For this review, take the finished solid that the model builds, in its own axes (mm). A direction names the side the tool comes from. Coordinates: 2 decimals unless noted, no trailing zeros. Write each loop counter-clockwise with the first axis right and the second up, starting at its lowest first coordinate (ties: lowest second). Pieces come first, ordered by that corner, then holes.
```python
from build123d import *

# Parameters (mm, degrees)
SKETCH_1_W          = 110
SKETCH_1_H          = 100
EXTRUDE_1_DEPTH     = 20
SKETCH_2_R          = 31.25
CUT_EXTRUDE_1_DEPTH = 14
SKETCH_3_R          = 21.5
CUT_EXTRUDE_2_DEPTH = 14
SKETCH_4_R          = 1.65
CUT_EXTRUDE_3_DEPTH = 77.974021592


with BuildPart() as part:
    # 草图1 → 凸台-拉伸1 (new body)
    with BuildSketch(Plane(origin=(0, 0, 0), x_dir=(0, 0, -1), z_dir=(1, 0, 0))):
        Rectangle(SKETCH_1_W, SKETCH_1_H)
    extrude(amount=EXTRUDE_1_DEPTH)

    # 草图2 → 切除-拉伸1 (cut)
    with BuildSketch(Plane(origin=(20, 0, 0), x_dir=(0, 0, -1), z_dir=(1, 0, 0))):
        Circle(SKETCH_2_R)
    extrude(amount=-CUT_EXTRUDE_1_DEPTH, mode=Mode.SUBTRACT)

    # 草图3 → 切除-拉伸2 (cut)
    with BuildSketch(Plane(origin=(6, 0, 0), x_dir=(0, 0, -1), z_dir=(1, 0, 0))):
        Circle(SKETCH_3_R)
    extrude(amount=-CUT_EXTRUDE_2_DEPTH, mode=Mode.SUBTRACT)

    # 草图4 → 切除-拉伸3 (cut, through all)
    with BuildSketch(Plane(origin=(20, 0, 0), x_dir=(0, 0, -1), z_dir=(1, 0, 0))):
        with Locations((33, 40)):
            Circle(SKETCH_4_R)
        with Locations((11, 40)):
            Circle(SKETCH_4_R)
        with Locations((-11, 40)):
            Circle(SKETCH_4_R)
        with Locations((-33, 40)):
            Circle(SKETCH_4_R)
        with Locations(Location((-11, -40, 0), (0, 0, 180))):
            Circle(SKETCH_4_R)
        with Locations(Location((11, -40, 0), (0, 0, 180))):
            Circle(SKETCH_4_R)
        with Locations(Location((33, -40, 0), (0, 0, 180))):
            Circle(SKETCH_4_R)
        with Locations(Location((-33, -40, 0), (0, 0, 180))):
            Circle(SKETCH_4_R)
    extrude(amount=-CUT_EXTRUDE_3_DEPTH, mode=Mode.SUBTRACT)


solid = part.part
```
1) Consider section A-A (z = 33). Give the boundary of the cut face in (x, y), then the cut area to 3 significant figures.
2) Consider section D-D (z = 0). Give the boundary of the cut face in (x, y), then the cut area to 3 significant figures.
3) Tool access review of faces 1 (the face through (10.14, 41.39, 10.11)), 2 (the face through (13.1, 1.37, 31.22)): name each direction out of +Z, -Z, +X, -X, +Y, -Y from which nothing blocks a thin tool from reaching the whole face with its end or side.
4) For L1, parallel to Y at x = 6.75, z = -33; L2, parallel to Y at x = 15.5, z = -11; L3, parallel to Y at x = 5.5, z = 12, list the stretches that pass through material, from the lowest coordinate up.
5) Clearance check with flat-ended pins moving along their axes: P1, Ø5.5, axis at y = -40, z = -11, coming from the +X side; P2, Ø2, axis at y = -8, z = 27, coming from the +X side; P3, Ø3, axis at y = 40, z = 11, coming from the +X side. State where each tip first meets the part, or that it passes through.
6) Consider section C-C (y = 0). Give the boundary of the cut face in (x, z), then the cut area to 3 significant figures.
7) The part is to be moulded in two halves that separate along Y. For faces 3 (the face through (10, -50, 1)), 4 (the face through (10, -1, 55)), 5 (the face through (10.14, -41.39, -10.11)), say which applies: pulls with the +Y half, pulls with the -Y half, needs draft (parallel to the pull), parting line crosses it, or undercut.
8) Consider section B-B (x = 4). Count the separate pieces of the cut face and the enclosed holes in it, then the cut area to 3 significant figures.
Results:
1. outline: (0, -50) - (20, -50) - (20, -41.65) - (0, -41.65) - close; (0, -38.35) - (20, -38.35) - (20, 38.35) - (0, 38.35) - close; (0, 41.65) - (20, 41.65) - (20, 50) - (0, 50) - close
1. area: 1,870 mm2
2. outline: (0, -50) - (20, -50) - (20, -31.25) - (6, -31.25) - (6, -21.5) - (0, -21.5) - close; (0, 21.5) - (6, 21.5) - (6, 31.25) - (20, 31.25) - (20, 50) - (0, 50) - close
2. area: 867 mm2
3. face 1: +X, -X
3. face 2: +X
4. L1: y = -50 to -41.65, -38.35 to 38.35, 41.65 to 50
4. L2: y = -50 to -41.65, -38.35 to -29.25, 29.25 to 38.35, 41.65 to 50
4. L3: y = -50 to -41.31, -38.69 to -17.84, 17.84 to 38.69, 41.31 to 50
5. P1: stops at x = 20
5. P2: stops at x = 6
5. P3: passes through
6. outline: (0, -55) - (20, -55) - (20, -31.25) - (6, -31.25) - (6, -21.5) - (0, -21.5) - close; (0, 21.5) - (6, 21.5) - (6, 31.25) - (20, 31.25) - (20, 55) - (0, 55) - close
6. area: 1,070 mm2
7. face 3: pulls with the -Y half
7. face 4: needs draft
7. face 5: undercut
8. separate pieces: 1
8. enclosed holes: 9
8. area: 9,480 mm2
